Can you work these out from the model? Positions are in its coordinate system, mm. A direction names the side the tool comes from. Give positions to 0.01 mm unless a question says otherwise; leave off trailing zeros. Loops run counter-clockwise (first coordinate to the right, second up) from the corner with the lowest first, then second, coordinate; pieces in that order, holes last. Notation, with made-up numbers: (-21, 57.25) - (29, 57.25) arc R29 ccw to (29, 96.25) - close; hole circle Ø3 at (-36.75, 31.5). An arc over 180 degrees is marked (long way). Answer as a JSON object with one key per item and string values.
```python
from build123d import *

# Parameters (mm, degrees)
SKETCH1_R           = 279.4
BOSS_EXTRUDE1_DEPTH = 609.6
CUT_EXTRUDE1_DEPTH  = 596.9
SKETCH4_R           = 12.7
BOSS_EXTRUDE2_DEPTH = 25.4


with BuildPart() as part:
    # Sketch1 → Boss-Extrude1 (new body)
    with BuildSketch(Plane(origin=(0, 0, 0), x_dir=(1, 0, 0), z_dir=(0, 1, 0))):
        Circle(SKETCH1_R)
    extrude(amount=BOSS_EXTRUDE1_DEPTH)

    # Sketch3 → Cut-Extrude1 (cut)
    with BuildSketch(Plane(origin=(0, 609.6, 0), x_dir=(1, 0, 0), z_dir=(0, 1, 0))):
        with BuildLine():
            ThreePointArc((127.809487072, 234.080381524), (-133.353402796, 230.967010551), (-266.624487569, 6.346071887))
            Line((-266.624487569, 6.346071887), (-3.672977901, 6.346071887))
            Line((-3.672977901, 6.346071887), (127.809487072, 234.080381524))
        make_face()
        with BuildLine():
            Line((-3.659370518, -6.353928113), (-266.624300463, -6.353928113))
            ThreePointArc((-266.624300463, -6.353928113), (-133.346597175, -230.970939778), (127.816384316, -234.07661545))
            Line((127.816384316, -234.07661545), (-3.659370518, -6.353928113))
        make_face()
        with BuildLine():
            ThreePointArc((266.7, 0), (232.539255974, 130.592436348), (138.808103253, 227.730543563))
            Line((138.808103253, 227.730543563), (7.332348419, 0.007856226))
            Line((7.332348419, 0.007856226), (138.814813391, -227.726453411))
            ThreePointArc((138.814813391, -227.726453411), (232.541179935, -130.589010389), (266.7, 0))
        make_face()
    extrude(amount=-CUT_EXTRUDE1_DEPTH, mode=Mode.SUBTRACT)

    # Sketch4 → Boss-Extrude2 (add)
    with BuildSketch(Plane.XZ):
        Circle(SKETCH4_R)
    extrude(amount=BOSS_EXTRUDE2_DEPTH)


solid = part.part
```
1) Which directions (+Z, -Z, +X, -X, +Y, -Y) give clear straight access to the entire face, cutting with the end or side of a thin tool? Please do faces 5 (the cylindrical face through (-130.031, 315.328, -232.854)), 6 (the cylindrical face through (-2.75, -12.52, -12.4)), 7 (the flat face through (-1, 609.6, -1)).
Check sheet entries:
{"face 5": "+Y", "face 6": "-Y", "face 7": "+Z, -Z, +X, -X, +Y"}
2) I'm going to push flat-ended pins straight in: P1, Ø1.5, axis at x = 44, y = 210.5, coming from the -Z side; P2, Ø12, axis at y = 38.5, z = -129.5, coming from the +X side; P3, Ø2, axis at y = 384.5, z = 147, coming from the -X side. Where does each tip first touch, or does it pass through?
Check sheet entries:
{"P1": "z = -276.03", "P2": "x = 250.62", "P3": "x = -238.22"}
3) If we mould it in two halves opening along X, with no side actions, what happens to faces 1 (the flat face through (-137, 315, -6.346)), 2 (the flat face through (135, 12.7, -3)), 3 (the cylindrical face through (-221.722, 300.533, 170.011)), 4 (the flat face through (0, -25.4, 0))? For each: released by +X, released by -X, zero draft, split by the parting line, or undercut.
Check sheet entries:
{"face 1": "undercut", "face 2": "undercut", "face 3": "split by the parting line", "face 4": "zero draft"}
4) Imagine slicing it at B-B on x = -168.5. Write out the boundary of the cut face in (y, z).
Check sheet entries:
{"outline": "(0, -222.87) - (609.6, -222.87) - (609.6, -206.73) - (12.7, -206.73) - (12.7, -6.35) - (609.6, -6.35) - (609.6, 6.35) - (12.7, 6.35) - (12.7, 206.73) - (609.6, 206.73) - (609.6, 222.87) - (0, 222.87) - close"}
5) I need wall thicknesses on L1, parallel to X at y = 536, z = -130; L2, parallel to Z at x = -181.5, y = 161; L3, parallel to X at y = 340.5, z = -41. Which ranges of each line are inside material? Lowest first, please.
Check sheet entries:
{"L1": "-247.31 to -232.87, 67.72 to 82.38, 232.87 to 247.31", "L2": "-212.42 to -195.41, -6.35 to 6.35, 195.41 to 212.42", "L3": "-276.38 to -263.53, 16.33 to 31, 263.53 to 276.38"}
6) Imagine slicing it at A-A on y = 272. Write out the boundary of the cut face in (x, z).
Check sheet entries:
{"outline": "circle Ø558.8 at (0, 0); hole (-266.62, -6.35) arc R266.7 ccw to (127.81, -234.08) - (-3.67, -6.35) - close; hole (-266.62, 6.35) - (-3.66, 6.35) - (127.82, 234.08) arc R266.7 ccw to start; hole (7.33, -0.01) - (138.81, -227.73) arc R266.7 ccw to (138.81, 227.73) - close"}
7) Imagine slicing it at D-D on x = 207.5. Write out the boundary of the cut face in (y, z), and give its area (3 significant figures).
Check sheet entries:
{"outline": "(0, -187.1) - (609.6, -187.1) - (609.6, -167.55) - (12.7, -167.55) - (12.7, 167.55) - (609.6, 167.55) - (609.6, 187.1) - (0, 187.1) - close", "area": "28,100 mm2"}
8) Imagine slicing it at C-C on z = 176.5. Write out the boundary of the cut face in (x, y).
Check sheet entries:
{"outline": "(-216.59, 0) - (216.59, 0) - (216.59, 609.6) - (199.94, 609.6) - (199.94, 12.7) - (109.24, 12.7) - (109.24, 609.6) - (94.57, 609.6) - (94.57, 12.7) - (-199.94, 12.7) - (-199.94, 609.6) - (-216.59, 609.6) - close"}
